Input: dimensioned drawing with shaded views. Units: mm. Origin: part minimum x, y, z. Round coordinates to 2 decimals unless told otherwise and drop trailing zeros. Order: outer loops, then holes, each group sorted by start corner. A loop starts at its lowest first (then second) coordinate and runs counter-clockwise, first axis right, second up. Notation, with made-up numbers: M 62,-18 L 97,-18 A21 cw 97,-6 Z; hole C -33.5,26 d10. An arc over 180 degrees is marked long. Put each result on its own line as item: value. Start each with the question number.
1) Section C-C, the plane z = 25. Return loops of the section in (x, y) (1 decimal), then the cut area to 3 significant figures.
2) Section D-D, the plane z = 42. Return loops of the section in (x, y), then the cut area to 3 significant figures.
3) Draft query along Z for the marked faces 1, 2, 3 and 4. Return one class per face: pulls with the +Z half, pulls with the -Z half, needs draft (parallel to the pull), parting line crosses it, or undercut.
4) Section B-B, the plane y = 14. Count the separate pieces of the cut face and the enclosed holes in it, then the cut area to 3 significant figures.
5) First-contact query: P1, Ø1, axis at x = 101, y = 22.5, coming from the +Z side (1 decimal); P2, Ø8, axis at x = 61.5, y = 28.5, coming from the +Z side (1 decimal); P3, Ø1, axis at y = 33, z = 41, coming from the +X side. Flat tips, straight axial feed; report the tip coordinate or a pass-through.
6) Section A-A, the plane x = 44.45. Return loops of the section in (y, z).
7) Material intervals for probe 1 along X at (y, z) = (34, 44); probe 2 along X at (y, z) = (29, 48) (1 decimal); probe 3 along Z at (x, y) = (76, 20), sorted ascending. Write a range as [from, to].
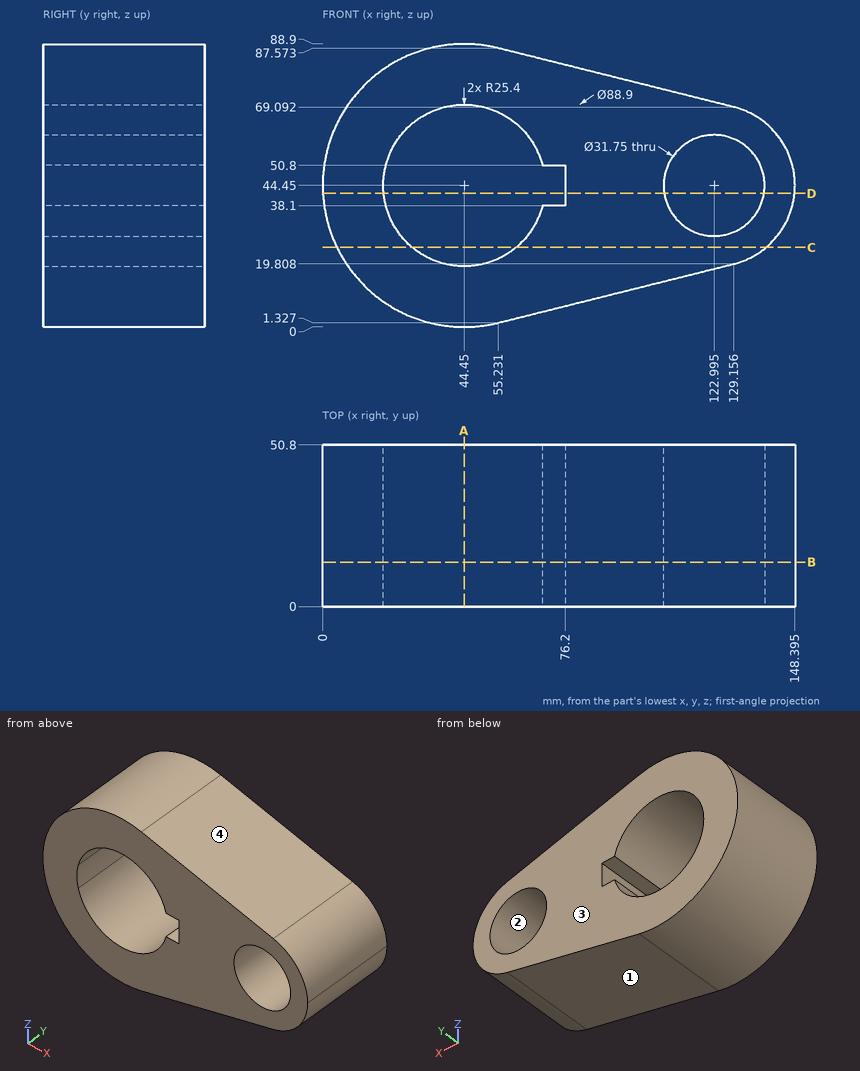
Result sheet:
1. outline: M 4.5,0 L 28.1,0 L 28.1,50.8 L 4.5,50.8 Z; M 60.8,0 L 139.3,0 L 139.3,50.8 L 60.8,50.8 Z
1. area: 5,190 mm2
2. outline: M 0.07,0 L 19.17,0 L 19.17,50.8 L 0.07,50.8 Z; M 76.2,0 L 107.31,0 L 107.31,50.8 L 76.2,50.8 Z; M 138.68,0 L 148.28,0 L 148.28,50.8 L 138.68,50.8 Z
2. area: 3,040 mm2
3. face 1: pulls with the -Z half
3. face 2: undercut
3. face 3: needs draft
3. face 4: pulls with the +Z half
4. separate pieces: 1
4. enclosed holes: 2
4. area: 6,860 mm2
5. P1: stops at z = 76.3
5. P2: stops at z = 87
5. P3: stops at x = 148.22
6. outline: M 0,0 L 50.8,0 L 50.8,19.05 L 0,19.05 Z; M 0,69.85 L 50.8,69.85 L 50.8,88.9 L 0,88.9 Z
7. probe 1: x = [0, 19.05], [76.2, 107.13], [138.86, 148.39]
7. probe 2: x = [0.1, 19.3], [76.2, 107.5], [138.5, 148.1]
7. probe 3: z = [6.52, 38.1], [50.8, 82.38]
